Study the drawing (mm; zero at the part's minimum x, y, z) and answer. A direction names the side the tool comes from. Give positions to 0.01 mm unless a question says otherwise; leave off trailing zeros. Loops run counter-clockwise (first coordinate to the right, second up) from the corner with the lowest first, then second, coordinate; pieces in that order, holes last. Notation, with made-up numbers: (1, -24.5) - (22, -24.5) arc R15 cw to (22, -20.5) - close; hole circle Ø1 at (-12.5, -3.5). An arc over 180 degrees is marked (long way). Write item = value, one per line. Start each with the question number.
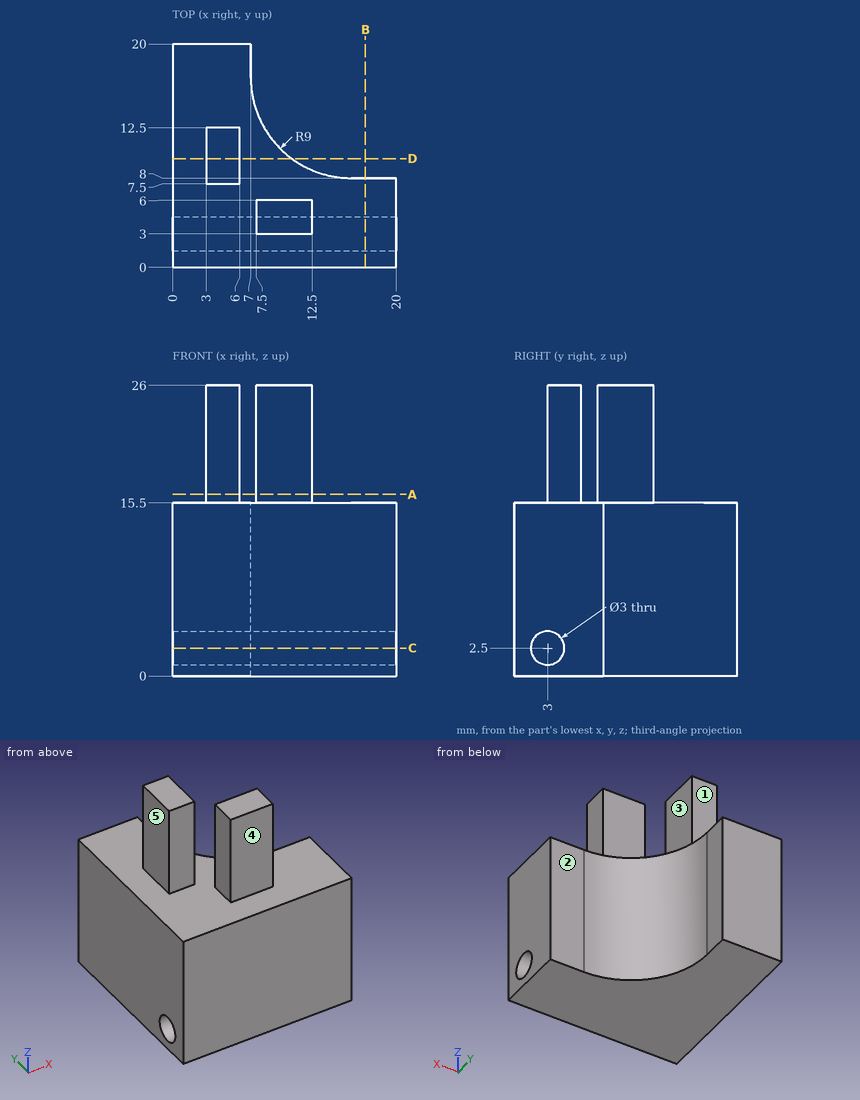
1. Consider line 1 along Z through (x, y) = (15, 3); line 2 along Y through (x, z) = (8, 23); line 3 along Z through (x, y) = (6.75, 6.5). Determine where each line is inside the solid, lowest interval first. Write a range as [from, to].
2. A cutting plane is placed at A-A on z = 16.25. Give the vertices of the cut face in (x, y).
3. A cutting plane is placed at B-B on x = 17.25. Give the vertices of the cut face in (y, z).
4. A cutting plane is placed at D-D on y = 9.75. Give the vertices of the cut face in (x, z), and give its area (3 significant figures).
5. A tool of negligible diameter and unlimited length cuts with its end or side. For the marked faces 1, 2, 3, 4 and 5, from which of +Z, -Z, +X, -X, +Y, -Y can it reach the whole face along a straight path? Write none if from no direction.
6. A cutting plane is placed at C-C on z = 2.5. Give the vertices of the cut face in (x, y), and give its area (3 significant figures).
7. Given P1, Ø1.5, axis at y = 4.5, z = 22.5, coming from the +X side; P2, Ø6, axis at x = 6, y = 17, coming from the +Z side; P3, Ø4, axis at y = 9, z = 22.5, coming from the -X side, each flat-ended and moving along its own axis, determine where each tip first touches the part or whether it passes through.
Reply:
q1.line_1 = [0, 1], [4, 15.5]
q1.line_2 = [3, 6]
q1.line_3 = [0, 15.5]
q2.outline = (3, 7.5) - (6, 7.5) - (6, 12.5) - (3, 12.5) - close; (7.5, 3) - (12.5, 3) - (12.5, 6) - (7.5, 6) - close
q3.outline = (0, 0) - (8, 0) - (8, 15.5) - (0, 15.5) - close; hole circle Ø3 at (3, 2.5)
q4.outline = (0, 0) - (10.67, 0) - (10.67, 15.5) - (6, 15.5) - (6, 26) - (3, 26) - (3, 15.5) - (0, 15.5) - close
q4.area = 197 mm^2
q5.face_1 = +Z, +X, -X, +Y
q5.face_2 = +Z, -Z, +X, +Y
q5.face_3 = +Z, +X, +Y, -Y
q5.face_4 = +Z, +X, -X, -Y
q5.face_5 = +Z, -X, +Y, -Y
q6.outline = (0, 0) - (20, 0) - (20, 1.5) - (0, 1.5) - close; (0, 4.5) - (20, 4.5) - (20, 8) - (16, 8) arc R9 cw to (7, 17) - (7, 20) - (0, 20) - close
q6.area = 201 mm^2
q7.P1 = 12.5
q7.P2 = 15.5
q7.P3 = 3
